from build123d import *

# Parameters (mm, degrees)
SKETCH1_W           = 75
SKETCH1_H           = 100
BOSS_EXTRUDE1_DEPTH = 10
SKETCH2_W           = 30
SKETCH2_H           = 58
SKETCH2_W_2         = 20
SKETCH2_H_2         = 40.9
BOSS_EXTRUDE2_DEPTH = 26.76
SKETCH3_R           = 2
CUT_EXTRUDE1_DEPTH  = 3
SKETCH4_R           = 2
CUT_EXTRUDE2_DEPTH  = 23


with BuildPart() as part:
    # Sketch1 → Boss-Extrude1 (new body)
    with BuildSketch(Plane(origin=(0, 0, 0), x_dir=(1, 0, 0), z_dir=(0, 1, 0))):
        Rectangle(SKETCH1_W, SKETCH1_H)
    extrude(amount=BOSS_EXTRUDE1_DEPTH)

    # Sketch2 → Boss-Extrude2 (add)
    with BuildSketch(Plane.XZ):
        with Locations((0, -11.900165179)):
            Rectangle(SKETCH2_W, SKETCH2_H)
        with Locations((0, -11.900165179)):
            Rectangle(SKETCH2_W_2, SKETCH2_H_2, mode=Mode.SUBTRACT)
    extrude(amount=BOSS_EXTRUDE2_DEPTH)

    # Sketch3 → Cut-Extrude1 (cut)
    with BuildSketch(Plane.XZ.offset(26.76)):
        with Locations(Location((-5, 12.399834821, 0), (0, 0, 270))):
            Circle(SKETCH3_R)
        with Locations(Location((5, 12.399834821, 0), (0, 0, 270))):
            Circle(SKETCH3_R)
        with Locations(Location((5, -36.200165179, 0), (0, 0, 270))):
            Circle(SKETCH3_R)
        with Locations(Location((-5, -36.200165179, 0), (0, 0, 270))):
            Circle(SKETCH3_R)
    extrude(amount=-CUT_EXTRUDE1_DEPTH, mode=Mode.SUBTRACT)

    # Sketch4 → Cut-Extrude2 (cut)
    with BuildSketch(Plane.XZ):
        with Locations(Location((-32.5, -45, 0), (0, 0, 270))):
            Circle(SKETCH4_R)
        with Locations(Location((32.5, -45, 0), (0, 0, 90))):
            Circle(SKETCH4_R)
        with Locations(Location((32.5, 45, 0), (0, 0, 270))):
            Circle(SKETCH4_R)
        with Locations(Location((-32.5, 45, 0), (0, 0, 90))):
            Circle(SKETCH4_R)
    extrude(amount=-CUT_EXTRUDE2_DEPTH, mode=Mode.SUBTRACT)


solid = part.part
The model under review builds one solid part; all positions refer to its coordinate system, in mm. A direction names the side the tool comes from. Give positions to 0.01 mm unless a question says otherwise; leave off trailing zeros. Write each loop counter-clockwise with the first axis right and the second up, starting at its lowest first coordinate (ties: lowest second). Pieces come first, ordered by that corner, then holes.
1. Add section D-D, the plane x = -13. Write out the cut boundary in (y, z), plus the area to 3 significant figures.
2. Add section A-A, the plane y = -1.5. Write out the cut boundary in (x, z).
3. Add section B-B, the plane x = -32.5. Write out the cut boundary in (y, z), plus the area to 3 significant figures.
4. Tool access review of faces 1 (the flat face through (-15, -13, -12)), 2 (the cylindrical face through (-30.548, 4.93, 44.566)), 3 (the flat face through (0, -13, 17.1)), 4 (the cylindrical face through (-4.912, -25.281, -34.202)): name each direction out of +Z, -Z, +X, -X, +Y, -Y from which nothing blocks a thin tool from reaching the whole face with its end or side.
5. Add section C-C, the plane z = -45. Write out the cut boundary in (x, y), plus the area to 3 significant figures.
6. For P1, Ø2, axis at x = -4.5, z = 13, coming from the -Y side; P2, Ø8, axis at y = -13.5, z = 2.5, coming from the +X side; P3, Ø6, axis at x = 3.5, y = -17.5, coming from the -Z side, all flat-tipped, find the tip position at first contact; note any pin that passes through.
7. Wall thickness on L1, parallel to X at y = 4, z = -45; L2, parallel to Z at x = -4, y = -8.5; L3, parallel to Z at x = -32, y = 3: over which ranges is each line inside the solid? List them lowest first.
8. Draft analysis for pull direction X (two halves, no side actions). For faces 5 (the flat face through (0, -13, -40.9)), 6 (the flat face through (0, 0, -12)), 7 (the flat face through (15, -13, -12)), state which applies: +X half, -X half, draft (parallel to the pull), parting line (faces both ways), or undercut.
Worked answers:
1. outline: (-26.76, -40.9) - (0, -40.9) - (0, -50) - (10, -50) - (10, 50) - (0, 50) - (0, 17.1) - (-26.76, 17.1) - close
1. area: 2,550 mm2
2. outline: (-15, -40.9) - (15, -40.9) - (15, 17.1) - (-15, 17.1) - close; hole (-10, -32.35) - (10, -32.35) - (10, 8.55) - (-10, 8.55) - close
3. outline: (0, -50) - (10, -50) - (10, -47) - (0, -47) - close; (0, -43) - (10, -43) - (10, 43) - (0, 43) - close; (0, 47) - (10, 47) - (10, 50) - (0, 50) - close
3. area: 920 mm2
4. face 1: +Z, -Z, -X, -Y
4. face 2: +Y, -Y
4. face 3: +Z, +X, -X, -Y
4. face 4: -Y
5. outline: (-37.5, 0) - (-34.5, 0) - (-34.5, 10) - (-37.5, 10) - close; (-30.5, 0) - (30.5, 0) - (30.5, 10) - (-30.5, 10) - close; (34.5, 0) - (37.5, 0) - (37.5, 10) - (34.5, 10) - close
5. area: 670 mm2
6. P1: stops at y = -23.76
6. P2: stops at x = 15
6. P3: stops at z = -40.9
7. L1: x = -37.5 to -34.5, -30.5 to 30.5, 34.5 to 37.5
7. L2: z = -40.9 to -32.35, 8.55 to 17.1
7. L3: z = -50 to -46.94, -43.06 to 43.06, 46.94 to 50
8. face 5: draft
8. face 6: undercut
8. face 7: +X half
